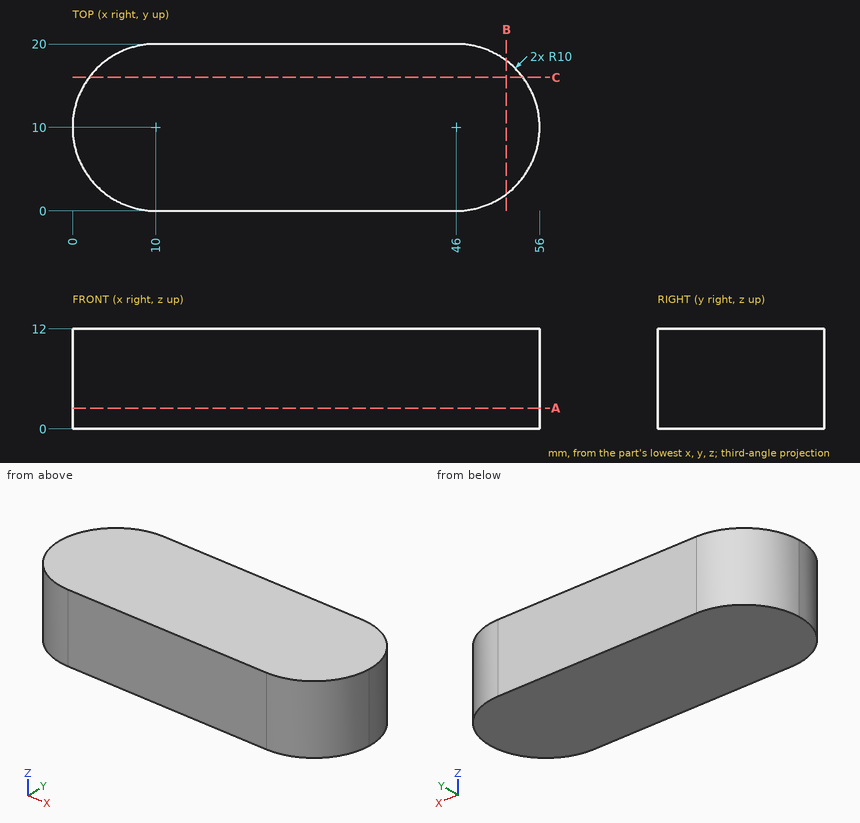
Source: three-view drawing plus pictorial views. Frame: mm from the lowest corner of the part. Round coordinates to 2 decimals unless told otherwise and drop trailing zeros. Loops run counter-clockwise (first coordinate to the right, second up) from the corner with the lowest first, then second, coordinate; pieces in that order, holes last.
1. Section query B-B on x = 52. Output: boundary loops of the cut face in (y, z).
2. Contact query for a flat-ended pin moving along its axis: pin 1 (5 mm diameter, centred on y = 6.5, z = 3, fed in from -X). Output: stop coordinate, or through.
3. Section query A-A on z = 2.5. Output: boundary loops of the cut face in (x, y).
4. Section query C-C on y = 16. Output: boundary loops of the cut face in (x, z), and give its area (3 significant figures).
5. Ray query, L1, parallel to X at y = 9.75, z = 5.75; L2, parallel to X at y = 11.5, z = 7.5; L3, parallel to Y at x = 51, z = 1.75. Return the intervals inside material, ascending.
Answers below:
1. outline: (2, 0) - (18, 0) - (18, 12) - (2, 12) - close
2. pin 1: stops at x = 0.05
3. outline: (0, 10) arc R10 ccw to (10, 0) - (46, 0) arc R10 ccw to (56, 10) arc R10 ccw to (46, 20) - (10, 20) arc R10 ccw to start
4. outline: (2, 0) - (54, 0) - (54, 12) - (2, 12) - close
4. area: 624 mm2
5. L1: x = 0 to 56
5. L2: x = 0.11 to 55.89
5. L3: y = 1.34 to 18.66
